Source: CAD feature listing. Evaluate the final solid. Frame: model axes, mm. A direction names the side the tool comes from. Coordinates: 2 decimals unless noted, no trailing zeros. Loops run counter-clockwise (first coordinate to the right, second up) from the corner with the lowest first, then second, coordinate; pieces in that order, holes last.
Item 1: Line query: probe 1 along X at (y, z) = (-3.5, 0); probe 2 along Z at (x, y) = (0, -7.5); probe 3 along Z at (x, y) = (0, -4.75). Output: solid intervals per line, ascending.
Item 2: Section query C-C, the plane z = 88.5. Return the cut outline in (x, y), then the cut area to 3 significant figures.
Item 3: Section query B-B, the plane z = 0. Return the cut outline in (x, y).
Item 4: Reachability of faces 1 (the flat face through (6.35, -6, 109)), 2 (the flat face through (2.54, -6, 197)), 3 (the flat face through (-6.35, -6, 109)) from +Z, -Z, +X, -X, +Y, -Y: full face, straight path, thin tool, end or side. Return the list, or none.
Item 5: Pull-direction query (Z, two-part tool) for faces 4 (the cylindrical face through (3.202, -6.261, 10.972)), 5 (the flat face through (0, -6, 203.2)), 6 (the flat face through (0, 0, 93)); classes: +Z half, -Z half, draft (parallel to the pull), parting line (faces both ways), or undercut.
Item 6: Section query A-A, the plane x = 0.25. Return the cut outline in (y, z) (3 decimals).
Item 7: Pin query (flat end, axial travel): pin 1 Ø5.5 at (y, z) = (-6.35, 196.85) entering from +X; pin 2 Ø5 at (y, z) = (-3, 69.5) entering from -X; pin 3 Ø12 at (x, z) = (-0.5, 92.5) entering from +Y; pin 4 Ø3 at (x, y) = (-2.5, -9.5) entering from -Z. Return the tip coordinate at first contact, or that it passes through.
```python
from build123d import *

# Parameters (mm, degrees)
F0_R          = 13.97
F0_R_2        = 11.43
F1_DEPTH      = 12.7
F2_W          = 12.7
F2_H          = 203.2
F3_DEPTH      = 6.35
F3_DEPTH_BACK = 6.35
F4_DEPTH      = 25.4
F6_START      = -3.81
F6_DEPTH      = 10.54779


with BuildPart() as f1:
    # F0 (on Front) → F1 (new body)
    with BuildSketch(Plane.XZ):
        Circle(F0_R)
        Circle(F0_R_2, mode=Mode.SUBTRACT)
    extrude(amount=F1_DEPTH)

    # F2 (on Right) → F3 (join, two sides)
    with BuildSketch(Plane.YZ) as f3_sk:
        with Locations((-6.35, 101.6)):
            Rectangle(F2_W, F2_H)
    extrude(amount=F3_DEPTH)
    extrude(f3_sk.sketch, amount=-F3_DEPTH_BACK)

    # F0 (on Front) → F4 (cut)
    with BuildSketch(Plane.XZ):
        Circle(F0_R_2)
    extrude(amount=F4_DEPTH, mode=Mode.SUBTRACT)

    # F5 (on face) → F6 (cut)
    with BuildSketch(Plane.YZ.offset(6.35).offset(F6_START)):
        with BuildLine():
            ThreePointArc((-3.175, 196.85), (-4.1049359697, 199.0950640303), (-6.35, 200.025))
            ThreePointArc((-6.35, 200.025), (-8.5950640303, 194.6049359697), (-3.175, 196.85))
        make_face()
    extrude(amount=-F6_DEPTH, mode=Mode.SUBTRACT)


solid = f1.part
```
Verdict:
1. probe 1: x = -13.97 to -11.43, 11.43 to 13.97
1. probe 2: z = -13.97 to -11.43, 11.43 to 193.89, 199.81 to 203.2
1. probe 3: z = -13.97 to -11.43, 11.43 to 194.11, 199.59 to 203.2
2. outline: (-6.35, -12.7) - (6.35, -12.7) - (6.35, 0) - (-6.35, 0) - close
2. area: 161 mm2
3. outline: (-13.97, -12.7) - (-11.43, -12.7) - (-11.43, 0) - (-13.97, 0) - close; (11.43, -12.7) - (13.97, -12.7) - (13.97, 0) - (11.43, 0) - close
4. face 1: +Z, +X, +Y, -Y
4. face 2: -X
4. face 3: +Z, -X, +Y, -Y
5. face 4: undercut
5. face 5: +Z half
5. face 6: draft
6. outline: (-12.7, -13.968) - (0, -13.968) - (0, -11.427) - (-12.7, -11.427) - close; (-12.7, 11.427) - (0, 11.427) - (0, 203.2) - (-12.7, 203.2) - close; hole circle Ø6.35 at (-6.35, 196.85)
7. pin 1: stops at x = 6.35
7. pin 2: stops at x = -6.35
7. pin 3: stops at y = 0
7. pin 4: stops at z = -13.93
